Geometry: final body of the model. Coordinates: model frame, mm. A direction names the side the tool comes from. Give positions to 0.01 mm unless a question says otherwise; leave off trailing zeros. Order: outer loops, then holes, each group sorted by start corner. A loop starts at its lowest first (then second) coordinate and runs counter-clockwise, first axis right, second up. Notation, with made-up numbers: (19.5, -36.75) - (50.5, -36.75) arc R15 cw to (50.5, -11.75) - close; hole circle Ø11 at (46, 23.5). An arc over 180 degrees is marked (long way). Use one line per item in the form item = value.
from build123d import *

# Parameters (mm, degrees)
SKETCH_1_W          = 200
SKETCH_1_H          = 400
EXTRUDE_1_DEPTH     = 8
SKETCH_2_R          = 60
CUT_EXTRUDE_1_DEPTH = 10
FILLET_1_R          = 60
SKETCH_5_R          = 4.25
CUT_EXTRUDE_4_DEPTH = 10
SKETCH_6_W          = 50
SKETCH_6_H          = 220
CUT_EXTRUDE_5_DEPTH = 10
FILLET_2_R          = 10
SKETCH_7_R          = 2.5
CUT_EXTRUDE_6_DEPTH = 69
SKETCH_8_R          = 6
CUT_EXTRUDE_7_DEPTH = 5.5
SKETCH_9_W          = 100
SKETCH_9_H          = 120
CUT_EXTRUDE_8_DEPTH = 10
FILLET_3_R          = 10


with BuildPart() as part:
    # 草图1 → 凸台-拉伸1 (new body)
    with BuildSketch(Plane.XY):
        with Locations((0, 200)):
            Rectangle(SKETCH_1_W, SKETCH_1_H)
    extrude(amount=EXTRUDE_1_DEPTH)

    # 草图2 → 切除-拉伸1 (cut)
    with BuildSketch(Plane(origin=(0, 0, 0), x_dir=(-1, 0, 0), z_dir=(0, 0, -1))):
        with Locations((0, 300)):
            Circle(SKETCH_2_R)
    extrude(amount=-CUT_EXTRUDE_1_DEPTH, mode=Mode.SUBTRACT)

    # 圆角1
    fillet_1_edges = [part.edges().sort_by_distance(p)[0] for p in [
        (100, 400, 4),
        (-100, 400, 4),
    ]]
    fillet(fillet_1_edges, radius=FILLET_1_R)

    # 草图5 → 切除-拉伸4 (cut)
    with BuildSketch(Plane(origin=(0, 0, 0), x_dir=(-1, 0, 0), z_dir=(0, 0, -1))):
        with Locations((-15, 25)):
            Circle(SKETCH_5_R)
        with Locations((15, 25)):
            Circle(SKETCH_5_R)
        with Locations((-15, 65)):
            Circle(SKETCH_5_R)
        with Locations((15, 65)):
            Circle(SKETCH_5_R)
        with Locations((-15, 175)):
            Circle(SKETCH_5_R)
        with Locations((15, 135)):
            Circle(SKETCH_5_R)
        with Locations((-15, 135)):
            Circle(SKETCH_5_R)
        with Locations((15, 175)):
            Circle(SKETCH_5_R)
    extrude(amount=-CUT_EXTRUDE_4_DEPTH, mode=Mode.SUBTRACT)

    # 草图6 → 切除-拉伸5 (cut)
    with BuildSketch(Plane(origin=(0, 0, 0), x_dir=(-1, 0, 0), z_dir=(0, 0, -1))):
        with Locations((75, 110)):
            Rectangle(SKETCH_6_W, SKETCH_6_H)
        with Locations((-75, 110)):
            Rectangle(SKETCH_6_W, SKETCH_6_H)
    extrude(amount=-CUT_EXTRUDE_5_DEPTH, mode=Mode.SUBTRACT)

    # 圆角2
    fillet_2_edges = [part.edges().sort_by_distance(p)[0] for p in [
        (-100, 220, 4),
        (-50, 220, 4),
        (100, 220, 4),
        (50, 220, 4),
    ]]
    fillet(fillet_2_edges, radius=FILLET_2_R)

    # 草图7 → 切除-拉伸6 (cut)
    with BuildSketch(Plane(origin=(0, 0, 0), x_dir=(-1, 0, 0), z_dir=(0, 0, -1))):
        with Locations((27.706208015, 376.380158009)):
            Circle(SKETCH_7_R)
        with Locations((52.294053173, 362.184358988)):
            Circle(SKETCH_7_R)
        with Locations((62.184358988, 352.294053173)):
            Circle(SKETCH_7_R)
        with Locations((76.380158009, 327.706208015)):
            Circle(SKETCH_7_R)
        with Locations((76.380158009, 272.293791985)):
            Circle(SKETCH_7_R)
        with Locations((62.184358988, 247.705946827)):
            Circle(SKETCH_7_R)
        with Locations((52.294053173, 237.815641012)):
            Circle(SKETCH_7_R)
        with Locations((27.706208015, 223.619841991)):
            Circle(SKETCH_7_R)
        with Locations((-27.706208015, 223.619841991)):
            Circle(SKETCH_7_R)
        with Locations((-52.294053173, 237.815641012)):
            Circle(SKETCH_7_R)
        with Locations((-62.184358988, 247.705946827)):
            Circle(SKETCH_7_R)
        with Locations((-76.380158009, 272.293791985)):
            Circle(SKETCH_7_R)
        with Locations((-76.380158009, 327.706208015)):
            Circle(SKETCH_7_R)
        with Locations((-62.184358988, 352.294053173)):
            Circle(SKETCH_7_R)
        with Locations((-52.294053173, 362.184358988)):
            Circle(SKETCH_7_R)
        with Locations((-27.706208015, 376.380158009)):
            Circle(SKETCH_7_R)
    extrude(amount=-CUT_EXTRUDE_6_DEPTH, mode=Mode.SUBTRACT)

    # 草图8 → 切除-拉伸7 (cut)
    with BuildSketch(Plane(origin=(0, 0, 0), x_dir=(-1, 0, 0), z_dir=(0, 0, -1))):
        with Locations((27.706208015, 376.380158009)):
            Circle(SKETCH_8_R)
        with Locations((52.294053173, 362.184358988)):
            Circle(SKETCH_8_R)
        with Locations((62.184358988, 352.294053173)):
            Circle(SKETCH_8_R)
        with Locations((76.380158009, 327.706208015)):
            Circle(SKETCH_8_R)
        with Locations((76.380158009, 272.293791985)):
            Circle(SKETCH_8_R)
        with Locations((62.184358988, 247.705946827)):
            Circle(SKETCH_8_R)
        with Locations((52.294053173, 237.815641012)):
            Circle(SKETCH_8_R)
        with Locations((27.706208015, 223.619841991)):
            Circle(SKETCH_8_R)
        with Locations((-27.706208015, 223.619841991)):
            Circle(SKETCH_8_R)
        with Locations((-52.294053173, 237.815641012)):
            Circle(SKETCH_8_R)
        with Locations((-62.184358988, 247.705946827)):
            Circle(SKETCH_8_R)
        with Locations((-76.380158009, 272.293791985)):
            Circle(SKETCH_8_R)
        with Locations((-76.380158009, 327.706208015)):
            Circle(SKETCH_8_R)
        with Locations((-62.184358988, 352.294053173)):
            Circle(SKETCH_8_R)
        with Locations((-52.294053173, 362.184358988)):
            Circle(SKETCH_8_R)
        with Locations((-27.706208015, 376.380158009)):
            Circle(SKETCH_8_R)
    extrude(amount=-CUT_EXTRUDE_7_DEPTH, mode=Mode.SUBTRACT)

    # 草图9 → 切除-拉伸8 (cut)
    with BuildSketch(Plane(origin=(0, 0, 0), x_dir=(-1, 0, 0), z_dir=(0, 0, -1))):
        with Locations((0, 60)):
            Rectangle(SKETCH_9_W, SKETCH_9_H)
    extrude(amount=-CUT_EXTRUDE_8_DEPTH, mode=Mode.SUBTRACT)

    # 圆角3
    fillet_3_edges = [part.edges().sort_by_distance(p)[0] for p in [
        (-50, 120, 4),
        (50, 120, 4),
    ]]
    fillet(fillet_3_edges, radius=FILLET_3_R)


solid = part.part
(1) Reachability of faces 5 (the face through (75, 220, 4)), 6 (the face through (-29, 221, 5.5)), 7 (the face through (-75, 220, 4)) from +Z, -Z, +X, -X, +Y, -Y: full face, straight path, thin tool, end or side. Return the list, or none.
Computed values:
face_5 = +Z, -Z, +X, -Y
face_6 = -Z
face_7 = +Z, -Z, -X, -Y
(2) Contact query for flat-ended pins moving along their axis: pin 1 Ø7 at (x, y) = (76.38, 327.71) entering from -Z; pin 2 Ø2 at (y, z) = (177, 6) entering from +X; pin 3 Ø1.5 at (x, z) = (53.5, 1) entering from +Y. Output: stop coordinate, or through.
Computed values:
pin_1 = 5.5
pin_2 = 50
pin_3 = 398.63
(3) Cut plane D-D on z = 3.75. Give the number of separate pieces and of enclosed holes in the cut face, plus the area to 3 significant figures.
Computed values:
separate_pieces = 1
enclosed_holes = 21
area = 31,100 mm²
(4) Cut plane A-A on y = 135. Output: boundary loops of the cut face in (x, z), plus the area to 3 significant figures.
Computed values:
outline = (-50, 0) - (-19.25, 0) - (-19.25, 8) - (-50, 8) - close; (-10.75, 0) - (10.75, 0) - (10.75, 8) - (-10.75, 8) - close; (19.25, 0) - (50, 0) - (50, 8) - (19.25, 8) - close
area = 664 mm²
(5) Cut plane B-B on y = 300. Output: boundary loops of the cut face in (x, z), plus the area to 3 significant figures.
Computed values:
outline = (-100, 0) - (-60, 0) - (-60, 8) - (-100, 8) - close; (60, 0) - (100, 0) - (100, 8) - (60, 8) - close
area = 640 mm²
(6) Cut plane C-C on x = 0. Output: boundary loops of the cut face in (y, z).
Computed values:
outline = (120, 0) - (240, 0) - (240, 8) - (120, 8) - close; (360, 0) - (400, 0) - (400, 8) - (360, 8) - close
(7) Ray query, line 1 along Y through (x, z) = (-23, 1.25); line 2 along Y through (x, z) = (32.5, 2.25); line 3 along X through (y, z) = (132.5, 5.5). Return the intervals inside material, ascending.
Computed values:
line_1 = 120 to 219.9, 227.34 to 244.58, 355.42 to 372.66, 380.1 to 400
line_2 = 120 to 220.01, 227.23 to 249.56, 350.44 to 372.77, 379.99 to 400
line_3 = -50 to -18.44, -11.56 to 11.56, 18.44 to 50
(8) Pull-direction query (X, two-part tool) for faces 1 (the face through (-14.447, 179.214, 3.944)), 2 (the face through (81.96, 382.89, 4.06)), 3 (the face through (25, 224, 5.5)), 4 (the face through (-82.89, 381.96, 4.06)); classes: released by +X, released by -X, zero draft, split by the parting line, or undercut.
Computed values:
face_1 = undercut
face_2 = released by +X
face_3 = undercut
face_4 = released by -X
